```python
from build123d import *

# Parameters (mm, degrees)
SKETCH1_W           = 8.6
SKETCH1_H           = 8.6
BOSS_EXTRUDE1_DEPTH = 3
CUT_EXTRUDE1_START  = 0.2
SKETCH1_14_R        = 1.1
CUT_EXTRUDE1_DEPTH  = 2.5
CUT_EXTRUDE2_START  = 0.2
SKETCH1_15_R        = 1.1
CUT_EXTRUDE2_DEPTH  = 2.8
BOSS_EXTRUDE2_START = -0.3
SKETCH2_W           = 7.8
SKETCH2_H           = 0.4
SKETCH2_W_2         = 0.4
SKETCH2_H_2         = 7.8
BOSS_EXTRUDE2_DEPTH = 0.1
CUT_EXTRUDE3_START  = -0.2
SKETCH3_W           = 0.6
SKETCH3_H           = 0.162741788
SKETCH3_H_2         = 0.6
CUT_EXTRUDE3_DEPTH  = 2


with BuildPart() as part:
    # Sketch1 → Boss-Extrude1 (new body)
    with BuildSketch(Plane(origin=(0, 0, 0), x_dir=(1, 0, 0), z_dir=(0, 1, 0))):
        with Locations((2.6, 2.6)):
            Rectangle(SKETCH1_W, SKETCH1_H)
    extrude(amount=BOSS_EXTRUDE1_DEPTH)

    # Sketch1<14> → Cut-Extrude1 (cut)
    with BuildSketch(Plane(origin=(0, 0, 0), x_dir=(1, 0, 0), z_dir=(0, 1, 0)).offset(CUT_EXTRUDE1_START)):
        Circle(SKETCH1_14_R)
        with BuildLine():
            Line((0, 1.1), (-1.7, 1.1))
            Line((-1.7, 1.1), (-1.7, -1.1))
            Line((-1.7, -1.1), (-0.1, -1.1))
            Line((-0.1, -1.1), (0, -1.1))
            ThreePointArc((0, -1.1), (-1.1, 0), (0, 1.1))
        make_face()
        with Locations((2.6, 0)):
            Circle(SKETCH1_14_R)
        with BuildLine():
            Line((1.5, -1.7), (3.7, -1.7))
            Line((3.7, -1.7), (3.7, 0))
            ThreePointArc((3.7, 0), (2.6, -1.1), (1.5, 0))
            Line((1.5, 0), (1.5, -1.7))
        make_face()
        with Locations((5.2, 0)):
            Circle(SKETCH1_14_R)
        with BuildLine():
            Line((6.9, -1.1), (6.9, 1.1))
            Line((6.9, 1.1), (5.2, 1.1))
            ThreePointArc((5.2, 1.1), (5.977817459, 0.777817459), (6.3, 0))
            ThreePointArc((6.3, 0), (5.977817459, -0.777817459), (5.2, -1.1))
            Line((5.2, -1.1), (6.9, -1.1))
        make_face()
        with BuildLine():
            Line((6.9, 1.5), (6.9, 3.7))
            Line((6.9, 3.7), (5.2, 3.7))
            ThreePointArc((5.2, 3.7), (5.977817459, 3.377817459), (6.3, 2.6))
            ThreePointArc((6.3, 2.6), (5.977817459, 1.822182541), (5.2, 1.5))
            Line((5.2, 1.5), (6.9, 1.5))
        make_face()
        with Locations((5.2, 2.6)):
            Circle(SKETCH1_14_R)
        with BuildLine():
            Line((6.9, 4.1), (6.9, 6.3))
            Line((6.9, 6.3), (5.2, 6.3))
            ThreePointArc((5.2, 6.3), (5.977817459, 5.977817459), (6.3, 5.2))
            ThreePointArc((6.3, 5.2), (5.977817459, 4.422182541), (5.2, 4.1))
            Line((5.2, 4.1), (6.9, 4.1))
        make_face()
        with Locations((5.2, 5.2)):
            Circle(SKETCH1_14_R)
        with BuildLine():
            Line((3.7, 5.2), (3.7, 6.9))
            Line((3.7, 6.9), (1.5, 6.9))
            Line((1.5, 6.9), (1.5, 5.2))
            ThreePointArc((1.5, 5.2), (2.6, 6.3), (3.7, 5.2))
        make_face()
        with Locations((2.6, 5.2)):
            Circle(SKETCH1_14_R)
        with Locations((0, 2.6)):
            Circle(SKETCH1_14_R)
        with BuildLine():
            Line((0, 3.7), (-1.7, 3.7))
            Line((-1.7, 3.7), (-1.7, 1.5))
            Line((-1.7, 1.5), (0, 1.5))
            ThreePointArc((0, 1.5), (-1.1, 2.6), (0, 3.7))
        make_face()
        with BuildLine():
            Line((-0.9, 6.3), (-1.7, 6.3))
            Line((-1.7, 6.3), (-1.7, 4.1))
            Line((-1.7, 4.1), (0, 4.1))
            ThreePointArc((0, 4.1), (-1.1, 5.2), (0, 6.3))
            Line((0, 6.3), (-0.9, 6.3))
        make_face()
        with Locations((0, 5.2)):
            Circle(SKETCH1_14_R)
    extrude(amount=CUT_EXTRUDE1_DEPTH, mode=Mode.SUBTRACT)

    # Sketch1<15> → Cut-Extrude2 (cut)
    with BuildSketch(Plane(origin=(0, 0, 0), x_dir=(1, 0, 0), z_dir=(0, 1, 0)).offset(CUT_EXTRUDE2_START)):
        with Locations(Location((2.6, 2.6, 0), (0, 0, 270))):
            Circle(SKETCH1_15_R)
    extrude(amount=CUT_EXTRUDE2_DEPTH, mode=Mode.SUBTRACT)

    # Sketch2 → Boss-Extrude2 (add)
    with BuildSketch(Plane.XZ.offset(BOSS_EXTRUDE2_START)):
        with Locations((2.6, 1.5)):
            Rectangle(SKETCH2_W, SKETCH2_H)
        with Locations((-1.5, -2.6)):
            Rectangle(SKETCH2_W_2, SKETCH2_H_2)
        with Locations((2.6, -6.7)):
            Rectangle(SKETCH2_W, SKETCH2_H)
        with Locations((6.7, -2.6)):
            Rectangle(SKETCH2_W_2, SKETCH2_H_2)
    extrude(amount=BOSS_EXTRUDE2_DEPTH)

    # Sketch3 → Cut-Extrude3 (cut)
    with BuildSketch(Plane.XZ.offset(CUT_EXTRUDE3_START)):
        Polygon((0.476549662, -0.03929145), (0.476549662, -0.591206698), (0.874813971, -0.246872241), (1.214094825, -0.63929145), (2.3, -0.63929145), (2.3, -0.476549662), (2.9, -0.476549662), (2.9, -0.63929145), (3.985905175, -0.63929145), (4.325186029, -0.246872241), (4.723450338, -0.591206698), (4.723450338, -0.03929145), align=None)
        with Locations((2.6, -0.557920556)):
            Rectangle(SKETCH3_W, SKETCH3_H)
        Polygon((0.874813971, -0.246872241), (0.476549662, -0.591206698), (0.476549662, -0.63929145), (1.214094825, -0.63929145), align=None)
        Polygon((4.325186029, -0.246872241), (3.985905175, -0.63929145), (4.723450338, -0.63929145), (4.723450338, -0.591206698), align=None)
        Polygon((3.343237824, -2.3), (2.9, -2.3), (2.9, -2.9), (3.304728308, -2.9), (4.723450338, -2.9), (4.723450338, -2.3), align=None)
        with Locations((2.6, -2.6)):
            Rectangle(SKETCH3_W, SKETCH3_H_2)
        Polygon((2.3, -2.3), (1.856762176, -2.3), (0.476549662, -2.3), (0.476549662, -2.9), (1.856762176, -2.9), (2.3, -2.9), align=None)
        Polygon((2.9, -2.9), (2.3, -2.9), (2.3, -3.304728308), (2.3, -4.56070855), (2.9, -4.56070855), (2.9, -3.343237824), align=None)
        Polygon((2.3, -1.895271692), (2.3, -2.3), (2.9, -2.3), (2.9, -1.895271692), (2.9, -0.63929145), (2.3, -0.63929145), align=None)
        with Locations((2.6, -4.642079444)):
            Rectangle(SKETCH3_W, SKETCH3_H)
        Polygon((2.3, -4.723450338), (2.3, -4.56070855), (1.214094825, -4.56070855), (0.874813971, -4.953127759), (0.476549662, -4.608793302), (0.476549662, -5.16070855), (4.723450338, -5.16070855), (4.723450338, -4.590835654), (4.56070855, -4.779066151), (4.308151662, -4.56070855), (2.9, -4.56070855), (2.9, -4.723450338), align=None)
        Polygon((0.874813971, -4.953127759), (1.214094825, -4.56070855), (0.476549662, -4.56070855), (0.476549662, -4.608793302), align=None)
        Polygon((4.723450338, -4.56070855), (4.308151662, -4.56070855), (4.56070855, -4.779066151), (4.723450338, -4.590835654), align=None)
    extrude(amount=-CUT_EXTRUDE3_DEPTH, mode=Mode.SUBTRACT)


solid = part.part
```
Model file for the job. Use its own axes, mm. A direction names the side the tool comes from. Coordinates: 2 decimals unless noted, no trailing zeros. Write each loop counter-clockwise with the first axis right and the second up, starting at its lowest first coordinate (ties: lowest second). Pieces come first, ordered by that corner, then holes. Notation, with made-up numbers: (52.5, -6) - (89.5, -6) arc R29 ccw to (89.5, 19) - close; hole circle Ø2 at (61, -12). An arc over 180 degrees is marked (long way). Use a Markdown table: item, result. Add a question column.
Item 1: Band-saw the part on A-A, the plane x = 2.6. Write the cut outline in (y, z), and give its area (3 significant figures).
Item 2: Band-saw the part on C-C, the plane x = 1.25. Write the cut outline in (y, z), and give its area (3 significant figures).
Item 3: Band-saw the part on D-D, the plane y = 1.55. Give the number of separate pieces and of enclosed holes in the cut face, and give its area (3 significant figures).
Item 4: Drill centre lines: line 1 along Z through (x, y) = (0, 0.7); line 2 along Z through (x, y) = (4, 0.25); line 3 along X through (y, z) = (2.3, -2.6). Where is each one in solid material? Low to high.
Item 5: Two-plate mould, pull along Z, no slides. Class faces 3 (the face through (6, 1, -3.7)), 4 (the face through (2, 3, -4)): pulls with the +Z half, pulls with the -Z half, needs draft (parallel to the pull), parting line crosses it, or undercut.
Item 6: 3-axis set-ups, long thin cutter, end or side, ignore diameter. For faces 1 (the face through (3, 0, -3)), 2 (the face through (5, 2.7, -5)): which of +Z, -Z, +X, -X, +Y, -Y reach the whole face in a straight line?
Item 7: Band-saw the part on B-B, the plane z = -1.25. Write the cut outline in (x, y).
A:
| question | item | result |
|---|---|---|
| 1 | outline | (0, -6.9) - (0.3, -6.9) - (0.3, -6.5) - (0.2, -6.5) - (0.2, 1.3) - (0.3, 1.3) - (0.3, 1.7) - (0, 1.7) - close; (2.2, -4.1) - (2.7, -4.1) - (2.7, -6.9) - (3, -6.9) - (3, -3.7) - (2.2, -3.7) - close; (2.2, -1.5) - (3, -1.5) - (3, 1.7) - (2.7, 1.7) - (2.7, -1.1) - (2.2, -1.1) - close |
| 1 | area | 4.12 mm² |
| 2 | outline | (0, -6.9) - (3, -6.9) - (3, 1.7) - (0, 1.7) - close; hole (0.2, -5.16) - (2.2, -5.16) - (2.2, -4.56) - (0.2, -4.56) - close; hole (0.2, -2.9) - (2.2, -2.9) - (2.2, -2.3) - (0.2, -2.3) - close; hole (0.2, -0.64) - (2.2, -0.64) - (2.2, -0.04) - (0.2, -0.04) - close |
| 2 | area | 22.2 mm² |
| 3 | separate pieces | 8 |
| 3 | enclosed holes | 0 |
| 3 | area | 22.7 mm² |
| 4 | line 1 | z = -6.9 to -6.3, -4.1 to -3.7, -1.5 to -1.1, 1.1 to 1.7 |
| 4 | line 2 | z = -6.9 to -5.16, -4.56 to -2.9, -2.3 to -0.64, -0.04 to 1.7 |
| 4 | line 3 | x = 1.1 to 1.5, 3.7 to 4.1 |
| 5 | face 3 | undercut |
| 5 | face 4 | needs draft |
| 6 | face 1 | +Z, -Z, +X, -X, -Y |
| 6 | face 2 | +X |
| 7 | outline | (-1.7, 0) - (6.9, 0) - (6.9, 3) - (-1.7, 3) - close; hole (2.3, 0.2) - (2.9, 0.2) - (2.9, 2.2) - (2.3, 2.2) - close |
